Work out the finished part from the listing and answer in its coordinate system (mm). Round coordinates to 2 decimals unless told otherwise and drop trailing zeros. Order: outer loops, then holes, each group sorted by start corner. A loop starts at its lowest first (then second) coordinate and runs counter-clockwise, first axis right, second up. Notation, with made-up numbers: M 29.25,55.25 L 44.25,55.25 A21 cw 44.25,67.25 Z; hole C -33.75,65.25 d4. An arc over 180 degrees is marked long. Return JSON: item names as keys, results as strings.
from build123d import *

# Parameters (mm, degrees)
F0_R     = 1.4
F1_DEPTH = 3.175


with BuildPart() as f1:
    # F0 (on Front) → F1 (new body)
    with BuildSketch(Plane.XZ):
        Polygon((9.525, -50.8), (47.625, -50.8), (47.625, -9.398), (50.8, -9.398), (50.8, 9.398), (47.625, 9.398), (47.625, 50.8), (9.525, 50.8), (9.525, 47.625), (1.4, 47.625), (1.4, 42.545), (3.125, 42.545), (3.125, 39.945), (1.4, 39.945), (1.4, 38.1), (-1.4, 38.1), (-1.4, 39.945), (-3.125, 39.945), (-3.125, 42.545), (-1.4, 42.545), (-1.4, 47.625), (-9.525, 47.625), (-9.525, 50.8), (-47.625, 50.8), (-47.625, 9.398), (-50.8, 9.398), (-50.8, -9.398), (-47.625, -9.398), (-47.625, -50.8), (-9.525, -50.8), (-9.525, -47.625), (-1.4, -47.625), (-1.4, -42.545), (-3.125, -42.545), (-3.125, -39.945), (-1.4, -39.945), (-1.4, -38.1), (1.4, -38.1), (1.4, -39.945), (3.125, -39.945), (3.125, -42.545), (1.4, -42.545), (1.4, -47.625), (9.525, -47.625), align=None)
        with Locations((-48.263, 0)):
            Circle(F0_R, mode=Mode.SUBTRACT)
        with Locations((48.263, 0)):
            Circle(F0_R, mode=Mode.SUBTRACT)
    extrude(amount=F1_DEPTH)


solid = f1.part
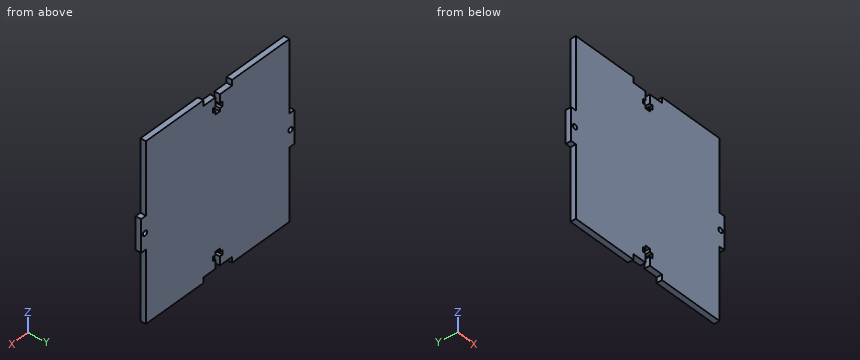
Item 1: Consider line 1 along X through (y, z) = (-0.5, -42) (3 decimals); line 2 along X through (y, z) = (-1.05, -45) (3 decimals); line 3 along X through (y, z) = (-2.15, -34.5) (3 decimals). Determine where each line is inside the solid, lowest interval first. Write a range as [from, to].
Output:
{"line 1": "x = [-47.625, -3.125], [3.125, 47.625]", "line 2": "x = [-47.625, -1.4], [1.4, 47.625]", "line 3": "x = [-47.625, 47.625]"}
Item 2: Each of these flat-tipped pins is pushed along its axis until it touches: pin 1 (1.9 mm diameter, centred on x = 2.5, y = -2, fed in from +Z) (3 decimals); pin 2 (1 mm diameter, centred on y = -1.5, z = 46, fed in from -X) (3 decimals); pin 3 (1.9 mm diameter, centred on x = -2, y = -1, fed in from -Z) (3 decimals). Where does it stop, or does it pass through?
Output:
{"pin 1": "stops at z = 47.625", "pin 2": "stops at x = -47.625", "pin 3": "stops at z = -47.625"}
Item 3: Find section C-C (y = -0.75). State how many separate pieces and enclosed holes the cut face has, plus the area to 3 significant figures.
Output:
{"separate pieces": "1", "enclosed holes": "2", "area": "9,590 mm^2"}
Item 4: Find section A-A (z = 0). Determine the outline of the cut face in (x, y) (3 decimals).
Output:
{"outline": "M -50.8,-3.175 L -49.663,-3.175 L -49.663,0 L -50.8,0 Z; M -46.863,-3.175 L 46.863,-3.175 L 46.863,0 L -46.863,0 Z; M 49.663,-3.175 L 50.8,-3.175 L 50.8,0 L 49.663,0 Z"}
Item 5: Find section B-B (z = 34). Determine the outline of the cut face in (x, y) (3 decimals).
Output:
{"outline": "M -47.625,-3.175 L 47.625,-3.175 L 47.625,0 L -47.625,0 Z"}
